Could you check a few things on this model? Use its own coordinates, in mm. Face numbers are marked on the shaded views. Coordinates: 2 decimals unless noted, no trailing zeros. Order: outer loops, then holes, each group sorted by start corner. A loop starts at its lowest first (then second) coordinate and runs counter-clockwise, first axis right, second up. Notation, with made-up numbers: (65.25, 44.5) - (104.25, 44.5) arc R22 cw to (104.25, 74.5) - close; hole circle Ø11 at (66, -22). An arc over 180 degrees is marked (long way). Answer as a JSON object with one key per item and string values. Group by question number.
(1) Imagine slicing it at B-B, the plane x = 72. Write out the boundary of the cut face in (y, z), and give its area (3 significant figures).
(2) Imagine slicing it at D-D, the plane x = 85.5. Write out the boundary of the cut face in (y, z).
(3) We'd pull the mould along X, two halves only. Please class the marked faces 1, 2, 3 and 4: pulls with the +X half, pulls with the -X half, needs draft (parallel to the pull), parting line crosses it, or undercut.
(4) Will these pins go through, and if not, where does the flat tip stop? P1, Ø2.5, axis at x = 81.57, y = 532.25, coming from the -Z side; P2, Ø5, axis at y = 524, z = 3301.5, coming from the +X side; P3, Ø3, axis at y = 518, z = 3305, coming from the +X side; P4, Ø5, axis at y = 514, z = 3301.5, coming from the -X side.
(5) Imagine slicing it at A-A, the plane y = 514.5. Write out the boundary of the cut face in (x, z), and give its area (3 significant figures).
(6) Please list where these lines run through material, in increasing order: probe 1 along Y at (x, z) = (81, 3303.25); probe 2 along Y at (x, z) = (80, 3298); probe 3 along X at (y, z) = (534, 3306).
(7) Imagine slicing it at C-C, the plane z = 3299.75. Write out the boundary of the cut face in (x, y).
from build123d import *

# Parameters (mm, degrees)
SKETCH2_R           = 4.25
SKETCH2_R_2         = 2.1
BOSS_EXTRUDE1_DEPTH = 10


with BuildPart() as part:
    # Sketch2 → Boss-Extrude1 (new body)
    with BuildSketch(Plane(origin=(0, 0, 3306.870187265), x_dir=(-1, 0, 0), z_dir=(0, 0, -1))):
        Polygon((-107.287132076, 528.630767378), (-87.295661635, 545.336840216), (-60.692285166, 513.501673478), (-80.683755608, 496.79560064), align=None)
        with Locations((-77.326966288, 511.582577545)):
            Circle(SKETCH2_R, mode=Mode.SUBTRACT)
        with Locations((-93.357902826, 530.766140137)):
            Circle(SKETCH2_R, mode=Mode.SUBTRACT)
        with Locations((-81.566936891, 532.251222865)):
            Circle(SKETCH2_R_2, mode=Mode.SUBTRACT)
        with Locations((-70.99449696, 519.599618719)):
            Circle(SKETCH2_R_2, mode=Mode.SUBTRACT)
    extrude(amount=BOSS_EXTRUDE1_DEPTH)


solid = part.part
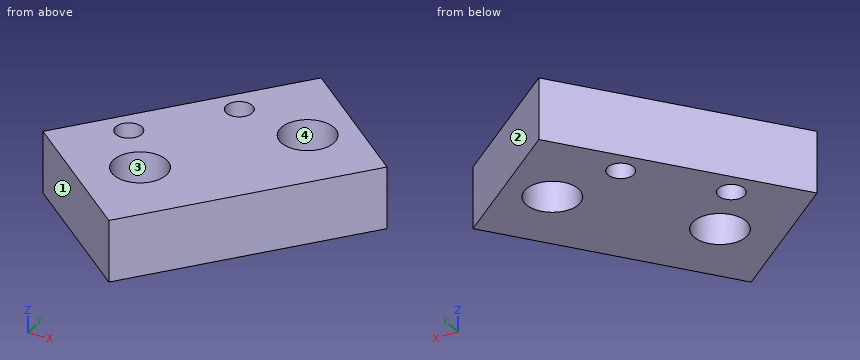
Result set:
{
 "1": {"outline": "(504.05, 3296.87) - (517.76, 3296.87) - (517.76, 3306.87) - (504.05, 3306.87) - close; (521.44, 3296.87) - (527.03, 3296.87) - (527.03, 3306.87) - (521.44, 3306.87) - close", "area": "193 mm^2"},
 "2": {"outline": "(502.56, 3296.87) - (543.19, 3296.87) - (543.19, 3306.87) - (502.56, 3306.87) - close"},
 "3": {"face 1": "pulls with the -X half", "face 2": "pulls with the +X half", "face 3": "undercut", "face 4": "undercut"},
 "4": {"P1": "passes through", "P2": "stops at x = 105.51", "P3": "stops at x = 99.66", "P4": "stops at x = 60.69"},
 "5": {"outline": "(61.53, 3296.87) - (74.24, 3296.87) - (74.24, 3306.87) - (61.53, 3306.87) - close; (80.42, 3296.87) - (95.48, 3296.87) - (95.48, 3306.87) - (80.42, 3306.87) - close", "area": "278 mm^2"},
 "6": {"probe 1": "y = 497.17 to 509.44, 513.72 to 530.23, 534.27 to 537.8", "probe 2": "y = 497.37 to 508.28, 514.89 to 530.85, 533.65 to 536.61", "probe 3": "x = 77.82 to 80.4, 82.73 to 90.6, 96.12 to 100.86"},
 "7": {"outline": "(60.69, 513.5) - (80.68, 496.8) - (107.29, 528.63) - (87.3, 545.34) - close; hole circle Ø4.2 at (70.99, 519.6); hole circle Ø8.5 at (77.33, 511.58); hole circle Ø4.2 at (81.57, 532.25); hole circle Ø8.5 at (93.36, 530.77)"}
}
